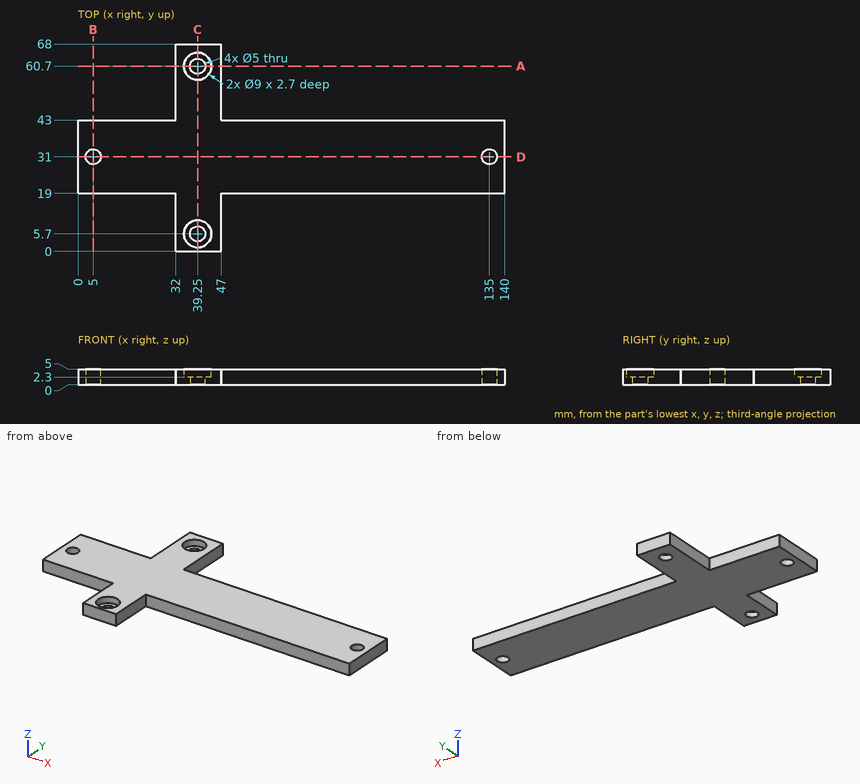
Check sheet for the drawn part. Datum: minimum x, y, z corner. Units: mm. Coordinates: 2 decimals unless noted, no trailing zeros. Order: outer loops, then holes, each group sorted by start corner. A loop starts at its lowest first (then second) coordinate and runs counter-clockwise, first axis right, second up. Notation, with made-up numbers: M 58.25,64.25 L 90.25,64.25 A18 cw 90.25,89.25 Z; hole C 5.5,25 d2. An arc over 180 degrees is marked long. One line per question, with ' | ' between items. Start each with the question number.
Item 1: Cross-section at A-A on y = 60.7. Enter the section's corners in (x, z), then the cut area to 3 significant figures.
Item 2: Cross-section at D-D on y = 31. Enter the section's corners in (x, z).
Item 3: Cross-section at B-B on x = 5. Enter the section's corners in (y, z), then the cut area to 3 significant figures.
Item 4: Material ranges on L1, parallel to Y at x = 39.25, z = 0.9; L2, parallel to X at y = 31, z = 4; L3, parallel to Y at x = 135, z = 3.85, recorded low to high. Write a range as [from, to].
Item 5: Gauge pin test, flat ends, axial feed: pin 1 (1.5 mm diameter, centred on x = 104.5, z = 3.5, fed in from -Y); pin 2 (1 mm diameter, centred on y = 44.5, z = 1, fed in from -X); pin 3 (6.5 mm diameter, centred on x = 39.25, y = 5.7, fed in from +Z). Record the tip position at first contact, or that the pin passes through.
Item 6: Cross-section at C-C on x = 39.25. Enter the section's corners in (y, z).
Findings:
1) outline: M 32,0 L 36.75,0 L 36.75,2.3 L 34.75,2.3 L 34.75,5 L 32,5 Z; M 41.75,0 L 47,0 L 47,5 L 43.75,5 L 43.75,2.3 L 41.75,2.3 Z | area: 39.2 mm²
2) outline: M 0,0 L 2.5,0 L 2.5,5 L 0,5 Z; M 7.5,0 L 132.5,0 L 132.5,5 L 7.5,5 Z; M 137.5,0 L 140,0 L 140,5 L 137.5,5 Z
3) outline: M 19,0 L 28.5,0 L 28.5,5 L 19,5 Z; M 33.5,0 L 43,0 L 43,5 L 33.5,5 Z | area: 95.0 mm²
4) L1: y = [0, 3.2], [8.2, 58.2], [63.2, 68] | L2: x = [0, 2.5], [7.5, 132.5], [137.5, 140] | L3: y = [19, 28.5], [33.5, 43]
5) pin 1: stops at y = 19 | pin 2: stops at x = 32 | pin 3: stops at z = 2.3
6) outline: M 0,0 L 3.2,0 L 3.2,2.3 L 1.2,2.3 L 1.2,5 L 0,5 Z; M 8.2,0 L 58.2,0 L 58.2,2.3 L 56.2,2.3 L 56.2,5 L 10.2,5 L 10.2,2.3 L 8.2,2.3 Z; M 63.2,0 L 68,0 L 68,5 L 65.2,5 L 65.2,2.3 L 63.2,2.3 Z
